```python
from build123d import *

# Parameters (mm, degrees)
BOSS_EXTRUDE1_DEPTH = 25
FILLET1_R           = 3
SKETCH2_R           = 2.2
CUT_EXTRUDE1_DEPTH  = 40


with BuildPart() as part:
    # Sketch1 → Boss-Extrude1 (new body)
    with BuildSketch(Plane.XY):
        Polygon((-24.6, 0), (24.6, 0), (24.6, 57), (27.6, 57), (27.6, -3), (9.6, -3), (9.6, -23), (6.6, -23), (6.6, -3), (-13.6, -3), (-13.6, -23), (-16.6, -23), (-16.6, -3), (-27.6, -3), (-27.6, 100), (-24.6, 100), align=None)
    extrude(amount=BOSS_EXTRUDE1_DEPTH)

    # Fillet1
    fillet1_edges = [part.edges().sort_by_distance(p)[0] for p in [
        (26.1, 57, 0),
        (8.1, -23, 0),
        (-15.1, -23, 0),
        (-15.1, -23, 25),
        (-26.1, 100, 0),
        (-24.6, 0, 12.5),
        (27.6, -3, 12.5),
        (9.6, -3, 12.5),
        (-16.6, -3, 12.5),
        (-27.6, -3, 12.5),
        (8.1, -23, 25),
        (26.1, 57, 25),
        (-26.1, 100, 25),
    ]]
    fillet(fillet1_edges, radius=FILLET1_R)

    # Sketch2 → Cut-Extrude1 (cut)
    with BuildSketch(Plane.ZY.offset(27.6)):
        with Locations(Location((12.5, 82, 0), (0, 0, 270))):
            Circle(SKETCH2_R)
        with Locations(Location((12.5, 32, 0), (0, 0, 270))):
            Circle(SKETCH2_R)
        with Locations(Location((12.5, -13, 0), (0, 0, 270))):
            Circle(SKETCH2_R)
    extrude(amount=-CUT_EXTRUDE1_DEPTH, mode=Mode.SUBTRACT)


solid = part.part
```
Input: part model. Units: mm. Frame: model coordinates. A direction names the side the tool comes from. Round coordinates to 2 decimals unless told otherwise and drop trailing zeros. Loops run counter-clockwise (first coordinate to the right, second up) from the corner with the lowest first, then second, coordinate; pieces in that order, holes last. Notation, with made-up numbers: (-7.5, -19.75) - (37.5, -19.75) arc R25 ccw to (37.5, 14.25) - close; hole circle Ø5 at (6, 48). An arc over 180 degrees is marked (long way). One line per item, written item: value. Start each with the question number.
(1) Section D-D, the plane y = -12.5. Return loops of the section in (x, z).
(2) Ray query, line 1 (Z direction, x = -26, y = 82); line 2 (X direction, y = 28.5, z = 20.5); line 3 (X direction, y = -16.5, z = 23). Return the intervals inside material, ascending. Write a range as [from, to].
(3) Contact query for flat-ended pins moving along their axis: P1, Ø13.5, axis at y = -11.5, z = 10, coming from the -X side; P2, Ø4, axis at y = -13, z = 12.5, coming from the +X side; P3, Ø1, axis at x = 5, z = 14.5, coming from the +Y side; P4, Ø6, axis at y = -13.5, z = 12, coming from the -X side. Output: stop coordinate, or through.
(4) Access query for faces 1 (the flat face through (-3, -3, 12)), 2 (the cylindrical face through (26.12, 56.14, 24.1)), 3 (the flat face through (19, -3, 12)), 4 (the flat face through (26, 57, 12)). Directions: +Z, -Z, +X, -X, +Y, -Y. A direction counts if a zero-diameter tool reaches every point of the face in a straight line with its end or side. Return the directions, or none.
(5) Section C-C, the plane y = 82. Return loops of the section in (x, z), plus the area to 3 significant figures.
(6) Section A-A, the plane y = 32. Return loops of the section in (x, z).
(7) Draft query along X for faces 5 (the flat face through (-16.6, -17, 12)), 6 (the cylindrical face through (-23.7, 0.86, 12.68)), 7 (the cylindrical face through (10.5, -3.86, 12.68)). Return one class per face: +X half, -X half, draft (parallel to the pull), parting line (faces both ways), or undercut.
(8) Section B-B, the plane z = 7. Return loops of the section in (x, y), plus the area to 3 significant figures.
Results below:
1. outline: (-16.6, 0) - (-13.6, 0) - (-13.6, 10.36) - (-16.6, 10.36) - close; (-16.6, 14.64) - (-13.6, 14.64) - (-13.6, 25) - (-16.6, 25) - close; (6.6, 0) - (9.6, 0) - (9.6, 10.36) - (6.6, 10.36) - close; (6.6, 14.64) - (9.6, 14.64) - (9.6, 25) - (6.6, 25) - close
2. line 1: [0, 10.3], [14.7, 25]
2. line 2: [-27.6, -24.6], [24.6, 27.6]
2. line 3: [-16.6, -13.6], [6.6, 9.6]
3. P1: x = -16.87
3. P2: through
3. P3: y = 0
3. P4: x = -16.6
4. face 1: +Z, -Z, -Y
4. face 2: +Z, +X, +Y
4. face 3: +Z, -Z, +X, -Y
4. face 4: +Z, -Z, +X, +Y
5. outline: (-27.6, 0) - (-24.6, 0) - (-24.6, 10.3) - (-27.6, 10.3) - close; (-27.6, 14.7) - (-24.6, 14.7) - (-24.6, 25) - (-27.6, 25) - close
5. area: 61.8 mm^2
6. outline: (-27.6, 0) - (-24.6, 0) - (-24.6, 10.3) - (-27.6, 10.3) - close; (-27.6, 14.7) - (-24.6, 14.7) - (-24.6, 25) - (-27.6, 25) - close; (24.6, 0) - (27.6, 0) - (27.6, 25) - (24.6, 25) - close
7. face 5: -X half
7. face 6: undercut
7. face 7: +X half
8. outline: (-27.6, 0) arc R3 ccw to (-24.6, -3) - (-19.6, -3) arc R3 cw to (-16.6, -6) - (-16.6, -23) - (-13.6, -23) - (-13.6, -3) - (6.6, -3) - (6.6, -23) - (9.6, -23) - (9.6, -6) arc R3 cw to (12.6, -3) - (24.6, -3) arc R3 ccw to (27.6, 0) - (27.6, 57) - (24.6, 57) - (24.6, 0) - (-21.6, 0) arc R3 cw to (-24.6, 3) - (-24.6, 100) - (-27.6, 100) - close
8. area: 759 mm^2
